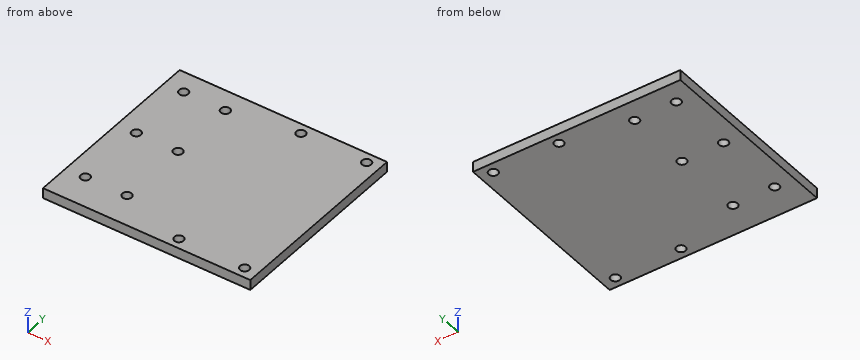
```python
from build123d import *

# Parameters (mm, degrees)
ESQUISSE1_W        = 101
ESQUISSE1_H        = 93
BOSS_EXTRU_1_DEPTH = 5
D_GAGEMENT_M41_D   = 4.5
D_GAGEMENT_M42_D   = 4.5


with BuildPart() as part:
    # Esquisse1 → Boss.-Extru.1 (new body)
    with BuildSketch(Plane.XY):
        Rectangle(ESQUISSE1_W, ESQUISSE1_H)
    extrude(amount=BOSS_EXTRU_1_DEPTH)

    # Dégagement M41 (through all)
    with Locations(Plane.XY.offset(5)):
        with Locations((44.157879946, 41.5), (12.157879946, 41.5), (12.157879946, -41.5), (44.157879946, -41.5)):
            Hole(D_GAGEMENT_M41_D / 2)

    # Dégagement M42 (through all)
    with Locations(Plane.XY.offset(5)):
        with Locations((-20.723129893, -30.91293976), (-20.723129893, 3.803464199), (-41.035821543, 3.803464199), (-41.035821543, -30.91293976), (-41.035821543, 35.983767161), (-20.723129893, 35.983767161)):
            Hole(D_GAGEMENT_M42_D / 2)


solid = part.part
```
Part model, mm, in its own coordinate system. Round coordinates to 2 decimals unless told otherwise and drop trailing zeros. Loops run counter-clockwise (first coordinate to the right, second up) from the corner with the lowest first, then second, coordinate; pieces in that order, holes last.
1. Slice it at A-A (y = 41.5). Give the cut face in (x, z), and give its area (3 significant figures).
Solutions:
outline: (-50.5, 0) - (9.91, 0) - (9.91, 5) - (-50.5, 5) - close; (14.41, 0) - (41.91, 0) - (41.91, 5) - (14.41, 5) - close; (46.41, 0) - (50.5, 0) - (50.5, 5) - (46.41, 5) - close
area: 460 mm2
2. Drill centre line: line 1 along X through (y, z) = (-31, 2.75). Where is it in solid material? Low to high.
Solutions:
line 1: x = -50.5 to -43.28, -38.79 to -22.97, -18.47 to 50.5
3. Slice it at B-B (z = 4). Count the separate pieces of the cut face and the enclosed holes in it, and give its area (3 significant figures).
Solutions:
separate pieces: 1
enclosed holes: 10
area: 9,230 mm2
4. Flat gauge pin, fed straight in: pin 1 (4 mm diameter, centred on x = 12.16, y = 41.5, fed in from -Z) (3 decimals). Where does the tip first touch, or does it go through?
Solutions:
pin 1: passes through
